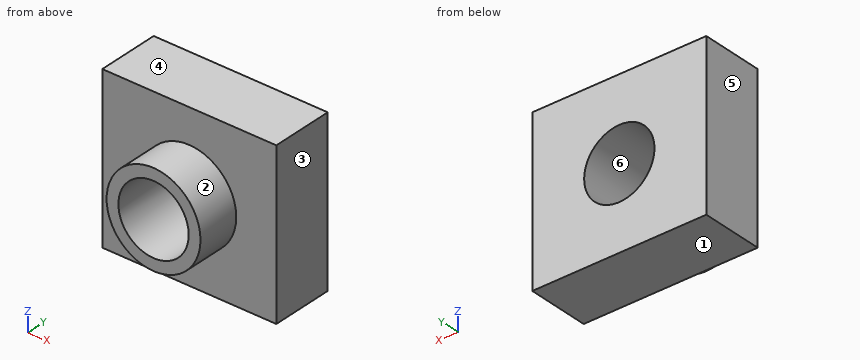
```python
from build123d import *

# Parameters (mm, degrees)
F0_W     = 102.1444201469
F0_H     = 95.3922867775
F1_DEPTH = 25.4
F2_R     = 27.5630659773
F4_DEPTH = 25.4
F5_R     = 20.638877023
F6_DEPTH = 50.801
F3_DEPTH = 11.1171808094


with BuildPart() as f1:
    # F0 (on Front) → F1 (new body)
    with BuildSketch(Plane.XZ):
        Rectangle(F0_W, F0_H)
    extrude(amount=F1_DEPTH)

    # F2 (on face) → F4 (join)
    with BuildSketch(Plane.XZ.offset(25.4)):
        Circle(F2_R)
    extrude(amount=F4_DEPTH)

    # F5 (on face) → F6 (cut, through all)
    with BuildSketch(Plane.XZ.offset(50.8)):
        Circle(F5_R)
    extrude(amount=-F6_DEPTH, mode=Mode.SUBTRACT)

    # F3 (add): a face of the model
    f3_faces = [f1.faces().sort_by_distance(p)[0] for p in [
        (0, 0, -46.2985321787),
    ]]
    extrude(f3_faces, amount=F3_DEPTH)


solid = f1.part
```
Here's how the part is built. I have some questions about the finished solid (model axes, mm). Face numbers are marked on the shaded views. A direction names the side the tool comes from. Give positions to 0.01 mm unless a question says otherwise; leave off trailing zeros. Loops run counter-clockwise (first coordinate to the right, second up) from the corner with the lowest first, then second, coordinate; pieces in that order, holes last. Notation, with made-up numbers: (9, 63) -> (35, 63) arc R26 ccw to (35, 91) -> close; hole circle Ø10 at (0, 65.25). An arc over 180 degrees is marked (long way). Use one line per item in the form item = value. Start each with the question number.
1) Imagine slicing it at B-B (z = 0). Please give me the cut outline in (x, y).
2) Which directions (+Z, -Z, +X, -X, +Y, -Y) give clear straight access to the entire face, cutting with the end or side of a thin tool? Please do the marked faces 1 and 2.
3) For P1, Ø1, axis at y = -41, z = -7.5, coming from the +X side; P2, Ø12, axis at x = -38, z = 34, coming from the -Y side; P3, Ø8, axis at x = -14.5, y = -35.5, coming from the -Z side, each with a flat end and sliding along its axis, tell me the tip position at first contact or that it passes through.
4) Please list where these lines run through material, in increasing order: line 1 along Z through (x, y) = (0, -37); line 2 along Y through (x, z) = (-44.5, 30); line 3 along Z through (x, y) = (0, -3).
5) Imagine slicing it at A-A (x = 0). Please give me the cut outline in (y, z), then the cut area to 3 significant figures.
6) Thinking about a two-plate mould opening in X: for the marked faces 3, 4, 5 and 6, which applies, +X half, -X half, draft (parallel to the pull), parting line (faces both ways), or undercut?
7) Imagine slicing it at D-D (x = 42). Please give me the cut outline in (y, z), then the cut area to 3 significant figures.
8) Imagine slicing it at C-C (y = -9.5). Please give me the cut outline in (x, z).
Check values:
q1.outline = (-51.07, -25.4) -> (-27.56, -25.4) -> (-27.56, -50.8) -> (-20.64, -50.8) -> (-20.64, 11.12) -> (-51.07, 11.12) -> close; (20.64, -50.8) -> (27.56, -50.8) -> (27.56, -25.4) -> (51.07, -25.4) -> (51.07, 11.12) -> (20.64, 11.12) -> close
q2.face_1 = -Z, +X, -X, +Y, -Y
q2.face_2 = -Y
q3.P1 = 26.66
q3.P2 = -25.4
q3.P3 = -25.48
q4.line_1 = -27.56 to -20.64, 20.64 to 27.56
q4.line_2 = -25.4 to 11.12
q4.line_3 = -47.7 to -20.64, 20.64 to 47.7
q5.outline = (-50.8, -27.56) -> (-25.4, -27.56) -> (-25.4, -47.7) -> (11.12, -47.7) -> (11.12, -20.64) -> (-50.8, -20.64) -> close; (-50.8, 20.64) -> (11.12, 20.64) -> (11.12, 47.7) -> (-25.4, 47.7) -> (-25.4, 27.56) -> (-50.8, 27.56) -> close
q5.area = 2,330 mm^2
q6.face_3 = +X half
q6.face_4 = draft
q6.face_5 = -X half
q6.face_6 = undercut
q7.outline = (-25.4, -47.7) -> (11.12, -47.7) -> (11.12, 47.7) -> (-25.4, 47.7) -> close
q7.area = 3,480 mm^2
q8.outline = (-51.07, -47.7) -> (51.07, -47.7) -> (51.07, 47.7) -> (-51.07, 47.7) -> close; hole circle Ø41.28 at (0, 0)
